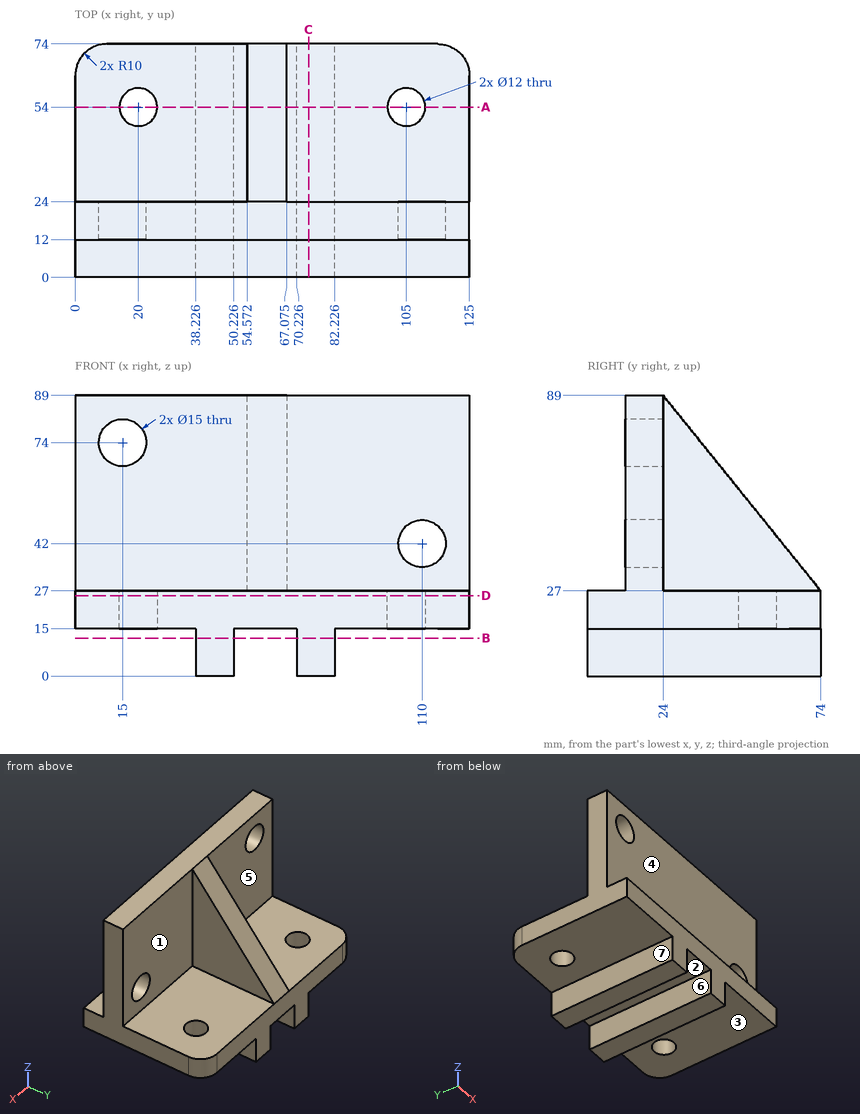
Geometry check sheet. Reference: drawing and pictorial views, mm from the part's lowest x, y, z. A direction names the side the tool comes from. Give positions to 0.01 mm unless a question says otherwise; leave off trailing zeros. Loops run counter-clockwise (first coordinate to the right, second up) from the corner with the lowest first, then second, coordinate; pieces in that order, holes last. Notation, with made-up numbers: M 82,42 L 130,42 A32 ccw 130,78 Z; hole C 28.25,83.5 d7. An arc over 180 degrees is marked long. Use a Markdown table: item, result. Add a question column.
Q1. Go/stop test with flat-tipped pins: pin 1 (24 mm diameter, centred on x = 110, z = 42, fed in from -Y); pin 2 (10 mm diameter, centred on y = 31, z = 43.5, fed in from -X); pin 3 (19 mm diameter, centred on x = 105, y = 54, fed in from -Z). Record where each tip stops, or that it passes through.
Q2. Scan lines: line 1 along X through (y, z) = (37, 13); line 2 along Y through (x, z) = (20, 24); line 3 along Z through (x, y) = (69, 21.5). Record each from-to range of solid material in increasing order. Write a range as [from, to].
Q3. Sectioned sample at D-D, the plane z = 25.5. Record the cut outline in (x, y), then the cut area to 3 significant figures.
Q4. Sectioned sample at C-C, the plane x = 74. Record the cut outline in (y, z).
Q5. Sectioned sample at B-B, the plane z = 12. Record the cut outline in (x, y).
Q6. Tool access check on the marked faces 1, 2, 3 and 4. Record the directions out of +Z, -Z, +X, -X, +Y, -Y that give a thin tool (end or side, any length) a straight path to the whole face; none if there is none.
Q7. Mould release check, pull along X, two halves, no side actions. Record for the marked faces 5, 6 and 7: pulls with the +X half, pulls with the -X half, needs draft (parallel to the pull), parting line crosses it, or undercut.
Q8. Sectioned sample at A-A, the plane y = 54. Record the cut outline in (x, z) (1 decimal), then the cut area to 3 significant figures.
Verdict:
| question | item | result |
|---|---|---|
| 1 | pin 1 | y = 12 |
| 1 | pin 2 | x = 54.57 |
| 1 | pin 3 | z = 15 |
| 2 | line 1 | [38.23, 50.23], [70.23, 82.23] |
| 2 | line 2 | [0, 48], [60, 74] |
| 2 | line 3 | [15, 89] |
| 3 | outline | M 0,0 L 125,0 L 125,64 A10 ccw 115,74 L 10,74 A10 ccw 0,64 Z; hole C 20,54 d12; hole C 105,54 d12 |
| 3 | area | 8,980 mm^2 |
| 4 | outline | M 0,0 L 74,0 L 74,27 L 24,27 L 24,89 L 12,89 L 12,27 L 0,27 Z |
| 5 | outline | M 38.23,0 L 50.23,0 L 50.23,74 L 38.23,74 Z; M 70.23,0 L 82.23,0 L 82.23,74 L 70.23,74 Z |
| 6 | face 1 | +Z, +X, +Y |
| 6 | face 2 | -Z, +Y, -Y |
| 6 | face 3 | -Z, +X, +Y, -Y |
| 6 | face 4 | +Z, +X, -X, -Y |
| 7 | face 5 | needs draft |
| 7 | face 6 | undercut |
| 7 | face 7 | pulls with the -X half |
| 8 | outline | M 0,15 L 14,15 L 14,27 L 0,27 Z; M 26,15 L 38.2,15 L 38.2,0 L 50.2,0 L 50.2,15 L 70.2,15 L 70.2,0 L 82.2,0 L 82.2,15 L 99,15 L 99,27 L 67.1,27 L 67.1,51.8 L 54.6,51.8 L 54.6,27 L 26,27 Z; M 111,15 L 125,15 L 125,27 L 111,27 Z |
| 8 | area | 1,880 mm^2 |
